Geometry: final body of the model. Coordinates: model frame, mm. Face numbers are marked on the shaded views. Give positions to 0.01 mm unless a question says otherwise; leave off trailing zeros. Order: outer loops, then holes, each group sorted by start corner. A loop starts at its lowest first (then second) coordinate and runs counter-clockwise, first axis right, second up. Notation, with made-up numbers: (-29, 65) - (17, 65) arc R38 cw to (17, 103) - close; hole circle Ø3 at (-6, -36.5). An arc over 180 degrees is marked (long way). One line per item, written item: value.
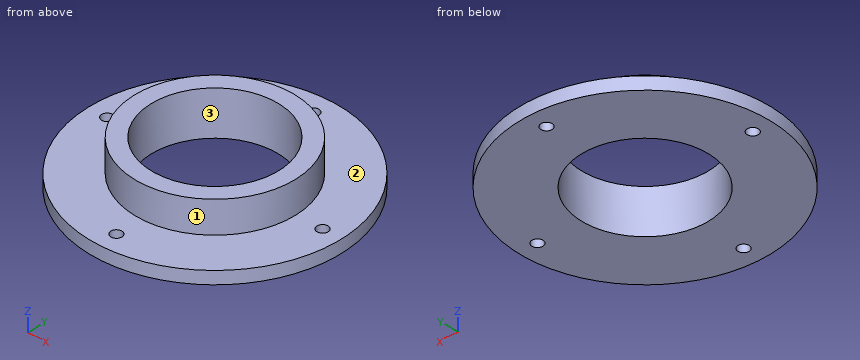
Autodesk Inventor part; units mm, degrees
ref_plane "YZ Plane" through (0, 0, 0) normal (1, 0, 0) x (0, 1, 0)
ref_plane "XZ Plane" through (0, 0, 0) normal (0, 1, 0) x (-1, 0, 0)
ref_plane "XY Plane" through (0, 0, 0) normal (0, 0, 1) x (1, 0, 0)
sketch "Sketch1" plane through (0, 0, 0) normal (0, 0, 1) x (1, 0, 0)
  circle A0 centre (0, 0) radius 25.2
  dimension "d0" = 50.4
extrude "Extrusion1" add sketch "Sketch1" along normal blind 10
sketch "Sketch2" plane through (0, 0, 10) normal (0, 0, 1) x (1, 0, 0)
  circle A0 centre (0, 0) radius 25.2
  circle A1 centre (0, 0) radius 7
  dimension "d3" = 14
extrude "Extrusion2" add sketch "Sketch2" along normal blind 6 contours A1
sketch "Sketch3" plane through (0, 0, 0) normal (0, 0, -1) x (-1, 0, 0)
  circle A0 centre (0, 0) radius 7
  circle A1 centre (0, 0) radius 39.5
  dimension "d6" = 79
extrude "Extrusion3" add sketch "Sketch3" along normal blind 4 contours A0 | A1
sketch "Sketch4" plane through (0, 0, 16) normal (0, 0, 1) x (1, 0, 0)
  circle A0 centre (0, 0) radius 7
  circle A1 centre (0, 0) radius 4
  dimension "d9" = 8
extrude "Extrusion4" cut sketch "Sketch4" against normal through all contours A1
sketch "Sketch5" plane through (0, 0, 0) normal (0, 0, 1) x (1, 0, 0)
  circle A0 centre (0, 0) radius 4
  line L0 (0, 0) -> (0, 39.5)
  circle A1 centre (0, 0) radius 39.5
  line L1 (0, 0) -> (0, -39.5)
  circle A2 centre (0, 0) radius 39.5
  circle A3 centre (0, 0) radius 4
  line L2 (0, 0) -> (38.7035, 0)
  circle A4 centre (0, 0) radius 7
  line L3 (0, 0) -> (-39.5, 0)
  circle A5 centre (0, 0) radius 7
  circle A6 centre (0, -33.5) radius 1.75
  circle A7 centre (33.5, 0) radius 1.75
  circle A8 centre (0, 33.5) radius 1.75
  circle A9 centre (-33.5, 0) radius 1.75
  circle A10 centre (0, 0) radius 33.5
  dimension "d13" = 3.5
  dimension "d19" = 67
extrude "Extrusion5" cut sketch "Sketch5" against normal through all contours A7 A10 L2 | L2 A10 A7 | A8 A10 L0 | L0 A10 A8 | A6 A10 L1 | L1 A10 A6 | A10 A7 L2 | L2 A7 A10 | A9 A10 L3 | L3 A10 A9 | A10 A8 L0 | L0 A8 A10 | A10 A6 L1 | L1 A6 A10 | A10 A9 L3 | L3 A9 A10
sketch "Sketch7" plane through (0, 0, -4) normal (0, 0, -1) x (-1, 0, 0)
  circle A0 centre (0, 0) radius 20
  dimension "d20" = 40
extrude "Extrusion7" cut sketch "Sketch7" against normal blind 75
properties part number "2209_Tube Flange_V1" material "ABS Plastic"
1) Section C-C, the plane z = -2. Return loops of the section in (x, y), then the cut area to 3 significant figures.
Answers below:
outline: circle Ø79 at (0, 0); hole circle Ø3.5 at (-33.5, 0); hole circle Ø40 at (0, 0); hole circle Ø3.5 at (0, -33.5); hole circle Ø3.5 at (0, 33.5); hole circle Ø3.5 at (33.5, 0)
area: 3,610 mm^2
2) Section D-D, the plane y = 33.5. Return loops of the section in (x, z).
Answers below:
outline: (-20.93, -4) - (-1.75, -4) - (-1.75, 0) - (-20.93, 0) - close; (1.75, -4) - (20.93, -4) - (20.93, 0) - (1.75, 0) - close
3) Material intervals for line 1 along Y through (x, z) = (0, -0.9); line 2 along Y through (x, z) = (-33.5, -1); line 3 along Y through (x, z) = (6, 4.75), sorted ascending.
Answers below:
line 1: -39.5 to -35.25, -31.75 to -20, 20 to 31.75, 35.25 to 39.5
line 2: -20.93 to -1.75, 1.75 to 20.93
line 3: -24.48 to -19.08, 19.08 to 24.48
4) Section A-A, the plane x = 0. Return loops of the section in (y, z), then the cut area to 3 significant figures.
Answers below:
outline: (-39.5, -4) - (-35.25, -4) - (-35.25, 0) - (-39.5, 0) - close; (-31.75, -4) - (-20, -4) - (-20, 10) - (-25.2, 10) - (-25.2, 0) - (-31.75, 0) - close; (20, -4) - (31.75, -4) - (31.75, 0) - (25.2, 0) - (25.2, 10) - (20, 10) - close; (35.25, -4) - (39.5, -4) - (39.5, 0) - (35.25, 0) - close
area: 232 mm^2
5) First-contact query: pin 1 (5 mm diameter, centred on y = -5, z = 0, fed in from -X); pin 2 (4 mm diameter, centred on x = 29, z = 1, fed in from +Y); pin 3 (5 mm diameter, centred on x = -8.5, z = 1, fed in from +Y). Flat tips, straight axial feed; report the tip coordinate or a pass-through.
Answers below:
pin 1: x = -39.42
pin 2: y = 28.58
pin 3: y = 39.01
6) Mould query, pull axis X, two halves, no side actions, for the marked faces 1, 2 and 3. Classes: released by +X, released by -X, zero draft, split by the parting line, or undercut.
Answers below:
face 1: split by the parting line
face 2: zero draft
face 3: undercut
